Autodesk Inventor part; units mm, degrees
ref_plane "YZ Plane" through (0, 0, 0) normal (1, 0, 0) x (0, 1, 0)
ref_plane "XZ Plane" through (0, 0, 0) normal (0, 1, 0) x (-1, 0, 0)
ref_plane "XY Plane" through (0, 0, 0) normal (0, 0, 1) x (1, 0, 0)
sketch "Sketch_1" plane through (0, 0, 0) normal (0, 0, 1) x (1, 0, 0)
  arc A0 (-12.7, -10.5664) -> (-10.5664, -12.7) centre (-10.592, -10.592) ccw
  arc A1 (-9.5504, -12.7) -> (-10.5664, -12.7) centre (-10.0584, -12.7) ccw
  line L0 (-9.5504, -12.7) -> (-6.3246, -12.7)
  arc A2 (-5.3086, -12.7) -> (-6.3246, -12.7) centre (-5.8166, -12.7) ccw
  line L1 (-5.3086, -12.7) -> (-4.3023, -12.7)
  arc A3 (-4.3023, -12.7) -> (-4.3023, -10.4902) centre (-4.3023, -11.5951) ccw
  line L2 (-4.3023, -10.4902) -> (-6.4748, -10.4902)
  arc A4 (-7.1932, -8.7558) -> (-6.4748, -10.4902) centre (-6.4748, -9.4742) ccw
  line L3 (-7.1932, -8.7558) -> (-3.8759, -5.4384)
  arc A5 (-1.6308, -4.5085) -> (-3.8759, -5.4384) centre (-1.6308, -7.6835) ccw
  line L4 (-1.6308, -4.5085) -> (1.6308, -4.5085)
  arc A6 (3.8759, -5.4384) -> (1.6308, -4.5085) centre (1.6308, -7.6835) ccw
  line L5 (3.8759, -5.4384) -> (7.1932, -8.7558)
  arc A7 (6.4748, -10.4902) -> (7.1932, -8.7558) centre (6.4748, -9.4742) ccw
  line L6 (6.4748, -10.4902) -> (4.3023, -10.4902)
  arc A8 (4.3023, -10.4902) -> (4.3023, -12.7) centre (4.3023, -11.5951) ccw
  line L7 (4.3023, -12.7) -> (5.3086, -12.7)
  arc A9 (6.3246, -12.7) -> (5.3086, -12.7) centre (5.8166, -12.7) ccw
  line L8 (6.3246, -12.7) -> (9.5504, -12.7)
  arc A10 (10.5664, -12.7) -> (9.5504, -12.7) centre (10.0584, -12.7) ccw
  arc A11 (10.5664, -12.7) -> (12.7, -10.5664) centre (10.592, -10.592) ccw
  arc A12 (12.7, -9.5504) -> (12.7, -10.5664) centre (12.7, -10.0584) ccw
  line L9 (12.7, -9.5504) -> (12.7, -6.3246)
  arc A13 (12.7, -5.3086) -> (12.7, -6.3246) centre (12.7, -5.8166) ccw
  line L10 (12.7, -5.3086) -> (12.7, -4.3023)
  arc A14 (12.7, -4.3023) -> (10.4902, -4.3023) centre (11.5951, -4.3023) ccw
  line L11 (10.4902, -4.3023) -> (10.4902, -6.4748)
  arc A15 (8.7558, -7.1932) -> (10.4902, -6.4748) centre (9.4742, -6.4748) ccw
  line L12 (8.7558, -7.1932) -> (5.4384, -3.8759)
  arc A16 (4.5085, -1.6308) -> (5.4384, -3.8759) centre (7.6835, -1.6308) ccw
  line L13 (4.5085, -1.6308) -> (4.5085, 1.6308)
  arc A17 (5.4384, 3.8759) -> (4.5085, 1.6308) centre (7.6835, 1.6308) ccw
  line L14 (5.4384, 3.8759) -> (8.7558, 7.1932)
  arc A18 (10.4902, 6.4748) -> (8.7558, 7.1932) centre (9.4742, 6.4748) ccw
  line L15 (10.4902, 6.4748) -> (10.4902, 4.3023)
  arc A19 (10.4902, 4.3023) -> (12.7, 4.3023) centre (11.5951, 4.3023) ccw
  line L16 (12.7, 4.3023) -> (12.7, 5.3086)
  arc A20 (12.7, 6.3246) -> (12.7, 5.3086) centre (12.7, 5.8166) ccw
  line L17 (12.7, 6.3246) -> (12.7, 9.5504)
  arc A21 (12.7, 10.5664) -> (12.7, 9.5504) centre (12.7, 10.0584) ccw
  arc A22 (12.7, 10.5664) -> (10.5664, 12.7) centre (10.592, 10.592) ccw
  arc A23 (9.5504, 12.7) -> (10.5664, 12.7) centre (10.0584, 12.7) ccw
  line L18 (9.5504, 12.7) -> (6.3246, 12.7)
  arc A24 (5.3086, 12.7) -> (6.3246, 12.7) centre (5.8166, 12.7) ccw
  line L19 (5.3086, 12.7) -> (4.3023, 12.7)
  arc A25 (4.3023, 12.7) -> (4.3023, 10.4902) centre (4.3023, 11.5951) ccw
  line L20 (4.3023, 10.4902) -> (6.4748, 10.4902)
  arc A26 (7.1932, 8.7558) -> (6.4748, 10.4902) centre (6.4748, 9.4742) ccw
  line L21 (7.1932, 8.7558) -> (3.8759, 5.4384)
  arc A27 (1.6308, 4.5085) -> (3.8759, 5.4384) centre (1.6308, 7.6835) ccw
  line L22 (1.6308, 4.5085) -> (-1.6308, 4.5085)
  arc A28 (-3.8759, 5.4384) -> (-1.6308, 4.5085) centre (-1.6308, 7.6835) ccw
  line L23 (-3.8759, 5.4384) -> (-7.1932, 8.7558)
  arc A29 (-6.4748, 10.4902) -> (-7.1932, 8.7558) centre (-6.4748, 9.4742) ccw
  line L24 (-6.4748, 10.4902) -> (-4.3023, 10.4902)
  arc A30 (-4.3023, 10.4902) -> (-4.3023, 12.7) centre (-4.3023, 11.5951) ccw
  line L25 (-4.3023, 12.7) -> (-5.3086, 12.7)
  arc A31 (-6.3246, 12.7) -> (-5.3086, 12.7) centre (-5.8166, 12.7) ccw
  line L26 (-6.3246, 12.7) -> (-9.5504, 12.7)
  arc A32 (-10.5664, 12.7) -> (-9.5504, 12.7) centre (-10.0584, 12.7) ccw
  arc A33 (-10.5664, 12.7) -> (-12.7, 10.5664) centre (-10.592, 10.592) ccw
  arc A34 (-12.7, 9.5504) -> (-12.7, 10.5664) centre (-12.7, 10.0584) ccw
  line L27 (-12.7, 9.5504) -> (-12.7, 6.3246)
  arc A35 (-12.7, 5.3086) -> (-12.7, 6.3246) centre (-12.7, 5.8166) ccw
  line L28 (-12.7, 5.3086) -> (-12.7, -5.3086)
  arc A36 (-12.7, -6.3246) -> (-12.7, -5.3086) centre (-12.7, -5.8166) ccw
  line L29 (-12.7, -6.3246) -> (-12.7, -9.5504)
  arc A37 (-12.7, -10.5664) -> (-12.7, -9.5504) centre (-12.7, -10.0584) ccw
  circle A38 centre (0, 0) radius 2.6035
  arc A39 (-10.4902, -6.4135) -> (-9.4742, -7.4295) centre (-9.4742, -6.4135) ccw
  arc A40 (-9.4742, -7.4295) -> (-8.6945, -7.1319) centre (-9.4638, -6.2865) ccw
  line L30 (-8.6945, -7.1319) -> (-5.4384, -3.8759)
  arc A41 (-5.4384, -3.8759) -> (-4.5085, -1.6308) centre (-7.6835, -1.6308) ccw
  line L31 (-4.5085, -1.6308) -> (-4.5085, 1.6308)
  arc A42 (-4.5085, 1.6308) -> (-5.4384, 3.8759) centre (-7.6835, 1.6308) ccw
  line L32 (-5.4384, 3.8759) -> (-8.6945, 7.1319)
  arc A43 (-8.6945, 7.1319) -> (-9.4742, 7.4295) centre (-9.4638, 6.2865) ccw
  arc A44 (-9.4742, 7.4295) -> (-10.4902, 6.4135) centre (-9.4742, 6.4135) ccw
  line L33 (-10.4902, 6.4135) -> (-10.4902, -6.4135)
extrude "Extrusion1" add sketch "Sketch_1" against normal blind 228.6
properties part number "1003-9-CL"
Geometry check sheet. Reference: the model listing, model coordinates, mm. Give positions to 0.01 mm unless a question says otherwise; leave off trailing zeros. Answer as a JSON object with one key per item and string values. Group by question number.
Item 1: Mould release check, pull along Y, two halves, no side actions. Record for faces 1 (the flat face through (-12.7, 0, -113)), 2 (the flat face through (-10.49, 0, -113)): pulls with the +Y half, pulls with the -Y half, needs draft (parallel to the pull), parting line crosses it, or undercut.
Item 2: Material ranges on L1, parallel to Y at x = 6.75, z = -178; L2, parallel to Y at x = -6.25, z = -186 (3 decimals); L3, parallel to Y at x = -3.5, z = -15, recorded low to high.
Item 3: Sectioned sample at A-A on z = -187.5. Give the number of separate pieces and of enclosed holes in the cut face, plus the area to 3 significant figures.
Item 4: Gauge pin test, flat ends, axial feed: pin 1 (1.6 mm diameter, centred on y = -0.5, z = -96.5, fed in from +X); pin 2 (1.5 mm diameter, centred on x = -1, z = -153, fed in from +Y); pin 3 (1.6 mm diameter, centred on x = -0.5, z = -98, fed in from -Y). Record the tip position at first contact, or that the pin passes through.
Findings below:
{
 "1": {"face 1": "needs draft", "face 2": "undercut"},
 "2": {"L1": "-12.7 to -10.45, -8.31 to -5.19, 5.19 to 8.31, 10.45 to 12.7", "L2": "-12.435 to -10.49, -7.813 to -4.687, 4.687 to 7.813, 10.49 to 12.435", "L3": "-12.35 to -10.84, -5.12 to 5.12, 10.84 to 12.35"},
 "3": {"separate pieces": "1", "enclosed holes": "2", "area": "296 mm2"},
 "4": {"pin 1": "x = 4.51", "pin 2": "y = 4.51", "pin 3": "y = -4.51"}
}
